Can you work these out from the model? Positions are in its coordinate system, mm. A direction names the side the tool comes from. Give positions to 0.01 mm unless a question says otherwise; leave off trailing zeros. Loops run counter-clockwise (first coordinate to the right, second up) from the corner with the lowest first, then second, coordinate; pieces in that order, holes last.
from build123d import *

# Parameters (mm, degrees)
F0_W     = 100
F0_H     = 100
F0_R     = 30
F1_DEPTH = 34
F2_R     = 50
F3_T     = -5


with BuildPart() as f1:
    # F0 (on Top) → F1 (new body)
    with BuildSketch(Plane.XY):
        Polygon((0, 100), (-50, 50), (50, 50), align=None)
        Rectangle(F0_W, F0_H)
        Circle(F0_R, mode=Mode.SUBTRACT)
    extrude(amount=F1_DEPTH)

    # F2
    f2_edges = [f1.edges().sort_by_distance(p)[0] for p in [
        (-50, 50, 17),
        (50, 50, 17),
    ]]
    fillet(f2_edges, radius=F2_R)

    # F3
    f3_openings = [f1.faces().sort_by_distance(p)[0] for p in [
        (-16.402915, 81.047576, 34),
    ]]
    offset(amount=F3_T, openings=f3_openings)


solid = f1.part
(1) Please list where these lines run through material, in increasing order: probe 1 along Y at (x, z) = (0, 15.5); probe 2 along Y at (x, z) = (-14, 19); probe 3 along X at (y, z) = (-5, 25.5).
Returned:
probe 1: y = -50 to -45, -35 to -30, 30 to 35, 92.93 to 100
probe 2: y = -50 to -45, -32.08 to -26.53, 26.53 to 32.08, 78.93 to 86
probe 3: x = -50 to -45, -34.64 to -29.58, 29.58 to 34.64, 45 to 50
(2) Thinking about a two-plate mould opening in X: for faces 3 (the cylindrical face through (46.088, 48.677, 17.238)), 4 (the flat face through (22, 26, 0)), 5 (the flat face through (-1, -45, 19)), 6 (the flat face through (-1, 40, 5)), which applies, pulls with the +X half, pulls with the -X half, needs draft (parallel to the pull), parting line crosses it, or undercut?
Returned:
face 3: pulls with the +X half
face 4: needs draft
face 5: undercut
face 6: undercut
(3) Which directions (+Z, -Z, +X, -X, +Y, -Y) give clear straight access to the entire face, cutting with the end or side of a thin tool? Please do faces 1 (the cylindrical face through (41.48, 46.74, 19.7)), 2 (the flat face through (50, -11, 17)).
Returned:
face 1: +Z
face 2: +Z, -Z, +X, +Y, -Y
(4) Suppose I cut it at A-A on y = 0. List the corners of the cut face in (x, z) for me, plus the area to 3 significant figures.
Returned:
outline: (-50, 0) - (-30, 0) - (-30, 34) - (-35, 34) - (-35, 5) - (-45, 5) - (-45, 34) - (-50, 34) - close; (30, 0) - (50, 0) - (50, 34) - (45, 34) - (45, 5) - (35, 5) - (35, 34) - (30, 34) - close
area: 780 mm2
(5) Suppose I cut it at B-B on z = 20.5. List the corners of the cut face in (x, y) for me, plus the area to 3 significant figures.
Returned:
outline: (-50, -50) - (50, -50) - (50, 29.29) arc R50 ccw to (35.36, 64.64) - (0, 100) - (-35.36, 64.64) arc R50 ccw to (-50, 29.29) - close; circle Ø70 at (0, 0); hole (-45, -45) - (45, -45) - (45, 29.29) arc R45 ccw to (31.82, 61.11) - (0, 92.93) - (-31.82, 61.11) arc R45 ccw to (-45, 29.29) - close; hole circle Ø60 at (0, 0)
area: 3,110 mm2
(6) Suppose I cut it at C-C on x = 13.5. List the corners of the cut face in (y, z) for me, plus the area to 3 significant figures.
Returned:
outline: (-50, 0) - (-26.79, 0) - (-26.79, 34) - (-32.29, 34) - (-32.29, 5) - (-45, 5) - (-45, 34) - (-50, 34) - close; (26.79, 0) - (86.5, 0) - (86.5, 34) - (79.43, 34) - (79.43, 5) - (32.29, 5) - (32.29, 34) - (26.79, 34) - close
area: 1,080 mm2
(7) Will these pins go through, and if not, where does the flat tip stop? P1, Ø1, axis at x = -36.5, y = -23.5, coming from the +Z side; P2, Ø10, axis at y = 72.5, z = 14.5, coming from the +X side; P3, Ø1.5, axis at x = 0, z = 13, coming from the +Y side.
Returned:
P1: stops at z = 5
P2: stops at x = 32.5
P3: stops at y = 100
